Geometry: final body of the model. Coordinates: model frame, mm. Give positions to 0.01 mm unless a question says otherwise; leave off trailing zeros. Write each loop counter-clockwise with the first axis right and the second up, starting at its lowest first coordinate (ties: lowest second). Pieces come first, ordered by that corner, then holes. Notation, with made-up numbers: M 17.25,-31 L 21.25,-31 A33 cw 21.25,6 Z; hole C 24,83.5 d1. An arc over 180 degrees is marked long. Answer as a JSON object with one key per item and string values.
from build123d import *

# Parameters (mm, degrees)
SKETCH1_W                      = 102.443759186
SKETCH1_H                      = 81.508386056
BOSS_EXTRUDE1_DEPTH            = 10
M5_CLEARANCE_HOLE1_D           = 5.5
M5_CLEARANCE_HOLE1_CSINK_D     = 5.55
M5_CLEARANCE_HOLE1_CSINK_ANGLE = 90
SKETCH5_R                      = 10
CUT_EXTRUDE1_DEPTH             = 67.216200422


with BuildPart() as part:
    # Sketch1 → Boss-Extrude1 (new body)
    with BuildSketch(Plane(origin=(0, 0, 0), x_dir=(1, 0, 0), z_dir=(0, 1, 0))):
        Rectangle(SKETCH1_W, SKETCH1_H)
    extrude(amount=BOSS_EXTRUDE1_DEPTH)

    # M5 Clearance Hole1 (through all)
    with Locations(Plane(origin=(0, 10, 0), x_dir=(1, 0, 0), z_dir=(0, 1, 0))):
        with Locations((-12.374368671, -12.374368671), (0, -17.5), (12.374368671, 12.374368671), (0, 17.5)):
            CounterSinkHole(M5_CLEARANCE_HOLE1_D / 2, M5_CLEARANCE_HOLE1_CSINK_D / 2, counter_sink_angle=M5_CLEARANCE_HOLE1_CSINK_ANGLE)

    # Sketch5 → Cut-Extrude1 (cut, through all)
    with BuildSketch(Plane(origin=(0, 10, 0), x_dir=(1, 0, 0), z_dir=(0, 1, 0))):
        with Locations(Location((0, 0, 0), (0, 0, 270))):
            Circle(SKETCH5_R)
    extrude(amount=-CUT_EXTRUDE1_DEPTH, mode=Mode.SUBTRACT)


solid = part.part
1) Cut plane B-B on x = 0. Return loops of the section in (y, z) (3 decimals), and give its area (3 significant figures).
Geometry check:
{"outline": "M 0,-40.754 L 10,-40.754 L 10,-20.275 L 9.975,-20.25 L 0,-20.25 Z; M 0,-14.75 L 9.975,-14.75 L 10,-14.725 L 10,-10 L 0,-10 Z; M 0,10 L 10,10 L 10,14.725 L 9.975,14.75 L 0,14.75 Z; M 0,20.25 L 9.975,20.25 L 10,20.275 L 10,40.754 L 0,40.754 Z", "area": "505 mm2"}
2) Line query: line 1 (X direction, y = 2.75, z = 0); line 2 (Z direction, x = 9, y = 6.5); line 3 (Z direction, x = -6, y = 6.25). Output: solid intervals per line, ascending. Write a range as from..to.
Geometry check:
{"line 1": "x = -51.22..-10, 10..51.22", "line 2": "z = -40.75..-4.36, 4.36..40.75", "line 3": "z = -40.75..-8, 8..40.75"}
3) Cut plane A-A on z = -8. Return loops of the section in (x, y), and give its area (3 significant figures).
Geometry check:
{"outline": "M -51.22,0 L -6,0 L -6,10 L -51.22,10 Z; M 6,0 L 51.22,0 L 51.22,10 L 6,10 Z", "area": "904 mm2"}
4) Cut plane D-D on z = 17.5. Return loops of the section in (x, y) (3 decimals), and give its area (3 significant figures).
Geometry check:
{"outline": "M -51.222,0 L -2.75,0 L -2.75,9.975 L -2.775,10 L -51.222,10 Z; M 2.75,0 L 51.222,0 L 51.222,10 L 2.775,10 L 2.75,9.975 Z", "area": "969 mm2"}
5) Cut plane C-C on y = 6.25. Return loops of the section in (x, z).
Geometry check:
{"outline": "M -51.22,-40.75 L 51.22,-40.75 L 51.22,40.75 L -51.22,40.75 Z; hole C -12.37,12.37 d5.5; hole C 0,0 d20; hole C 0,-17.5 d5.5; hole C 0,17.5 d5.5; hole C 12.37,-12.37 d5.5"}
6) Pull-direction query (Z, two-part tool) for faces 1 (the cylindrical face through (0.358, 4.918, -20.227)), 2 (the flat face through (-1, 5, 40.754)), 3 (the cylindrical face through (-9.76, 5.07, -2.17)), 4 (the flat face through (51.222, 5, 1)); classes: pulls with the +Z half, pulls with the -Z half, needs draft (parallel to the pull), parting line crosses it, or undercut.
Geometry check:
{"face 1": "undercut", "face 2": "pulls with the +Z half", "face 3": "undercut", "face 4": "needs draft"}
